The drawing under review shows one solid part. Ordinate dimensions are in mm from its lowest x, y, z. A direction names the side the tool comes from. Round coordinates to 2 decimals unless told otherwise and drop trailing zeros. Write each loop counter-clockwise with the first axis right and the second up, starting at its lowest first coordinate (ties: lowest second). Pieces come first, ordered by that corner, then holes.
Item 1: To check wall thickness, follow L1, parallel to Z at x = 5, y = 3.4; L2, parallel to Y at x = 6.75, z = 5; L3, parallel to X at y = 4.5, z = 3.75. State the ranges of each line that lie inside material, in increasing order.
Item 2: Clearance check with flat-ended pins moving along their axes: pin 1 Ø3 at (y, z) = (4, 5) entering from -X; pin 2 Ø1.5 at (x, z) = (5, 9) entering from -Y; pin 3 Ø1.8 at (x, z) = (4, 3.5) entering from -Y; pin 4 Ø1.5 at (y, z) = (2, 9) entering from +X. State where each tip first meets the part, or that it passes through.
Item 3: Add section C-C (z = 1.5). Give the boundary of the cut face in (x, y).
Item 4: Add section B-B (y = 0.5). Give the boundary of the cut face in (x, z).
Item 5: Add section D-D (x = 7). Give the boundary of the cut face in (y, z).
Item 6: Add section A-A (x = 5). Give the boundary of the cut face in (y, z).
Item 7: Machinability: for the marked faces 4, 5 and 6, which of the approach directions +Z, -Z, +X, -X, +Y, -Y give a long, thin tool a straight path to every point of the face, cutting with its end or side? Answer none if there is none.
Item 8: Draft analysis for pull direction Z (two halves, no side actions). For the marked faces 1, 2 and 3, state which applies: +Z half, -Z half, draft (parallel to the pull), parting line (faces both ways), or undercut.
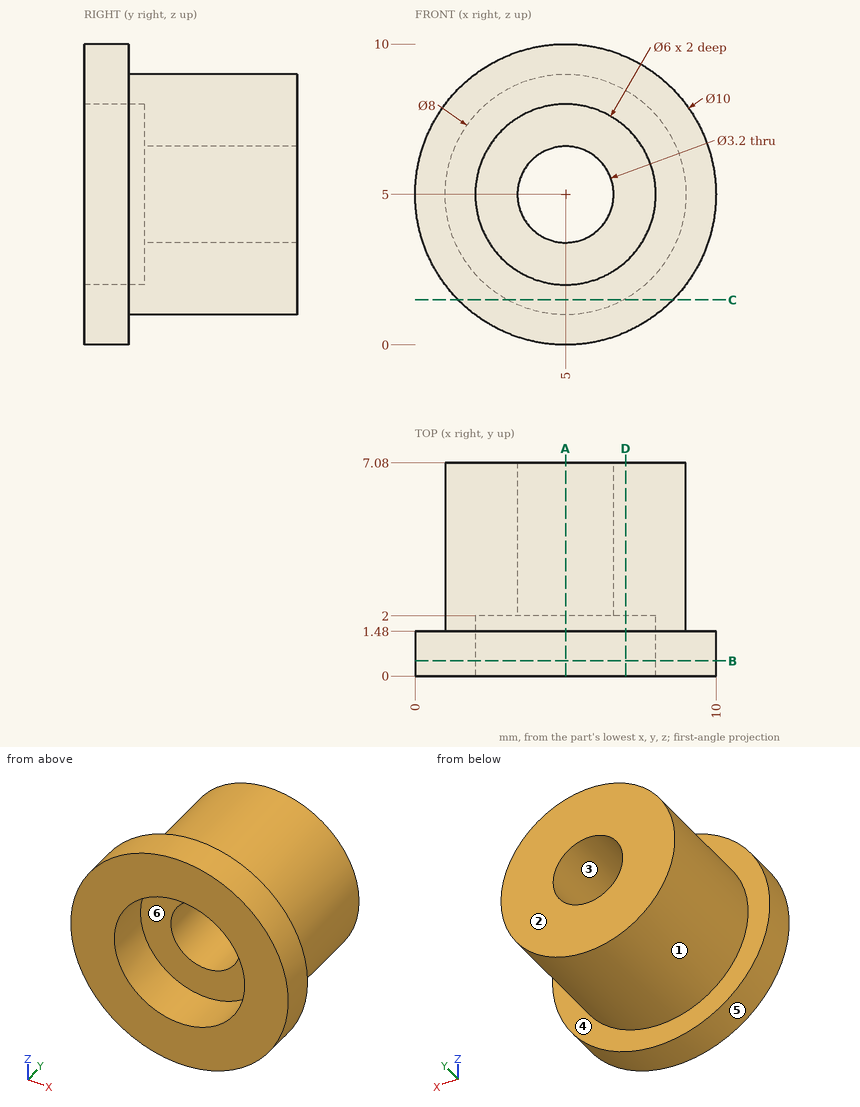
Numbers:
1. L1: z = 1 to 3.4, 6.6 to 9
1. L2: y = 2 to 7.08
1. L3: x = 1.2 to 4, 6 to 8.8
2. pin 1: stops at x = 1
2. pin 2: stops at y = 0
2. pin 3: stops at y = 2
2. pin 4: stops at x = 8.61
3. outline: (1.43, 0) - (8.57, 0) - (8.57, 1.48) - (6.94, 1.48) - (6.94, 7.08) - (3.06, 7.08) - (3.06, 1.48) - (1.43, 1.48) - close
4. outline: circle Ø10 at (5, 5); hole circle Ø6 at (5, 5)
5. outline: (0, 0.42) - (1.48, 0.42) - (1.48, 1.54) - (7.08, 1.54) - (7.08, 8.46) - (1.48, 8.46) - (1.48, 9.58) - (0, 9.58) - (0, 7.24) - (2, 7.24) - (2, 2.76) - (0, 2.76) - close
6. outline: (0, 0) - (1.48, 0) - (1.48, 1) - (7.08, 1) - (7.08, 3.4) - (2, 3.4) - (2, 2) - (0, 2) - close; (0, 8) - (2, 8) - (2, 6.6) - (7.08, 6.6) - (7.08, 9) - (1.48, 9) - (1.48, 10) - (0, 10) - close
7. face 4: +Y
7. face 5: +Y, -Y
7. face 6: -Y
8. face 1: parting line
8. face 2: draft
8. face 3: undercut
